Design review of the part built by this model. Coordinates are the model's own, in mm. A direction names the side the tool comes from. Coordinates: 2 decimals unless noted, no trailing zeros. One line per question, with ' | ' between items.
from build123d import *

# Parameters (mm, degrees)
SHELL1_T                                = -2.54
CUT_EXTRUDE2_DEPTH                      = 38.003022678
CIRPATTERN1_COUNT                       = 2
CIRPATTERN1_ANGLE                       = 90
BOSS_EXTRUDE3_DEPTH                     = 6.985
BOSS_EXTRUDE3_DEPTH_BACK                = 2.54
SKETCH13_R                              = 8.663884536
CBORE_FOR_M5_HEX_HEAD_BOLT2_D           = 4.5
CBORE_FOR_M5_HEX_HEAD_BOLT2_CBORE_D     = 7.5
CBORE_FOR_M5_HEX_HEAD_BOLT2_CBORE_DEPTH = 4


with BuildPart() as part:
    # Sketch1 → Revolve1 (revolve)
    with BuildSketch(Plane.XY, mode=Mode.PRIVATE) as revolve1_sk:
        with BuildLine():
            Line((0, 23.722851324), (5.5245, 23.722851324))
            ThreePointArc((5.5245, 23.722851324), (9.236535333, 23.238492745), (12.7, 21.817851324))
            Line((12.7, 21.817851324), (12.7, 20.547851324))
            Line((12.7, 20.547851324), (8.89, 20.547851324))
            add(Edge.make_bspline(
                [(8.89, 20.547851324), (8.84961008, 12.497906194), (9.741228483, 4.469234919), (9.525, -3.582148676)],
                knots=[0, 0, 0, 0, 1, 1, 1, 1], degree=3))
            Line((9.525, -3.582148676), (0, -3.582148676))
            Line((0, -3.582148676), (0, 23.722851324))
        make_face()
    revolve(revolve1_sk.sketch.rotate(Axis((0, 23.722851324, 0), (0, -1, 0)), 180), axis=Axis((0, 23.722851324, 0), (0, -1, 0)))

    # Shell1
    shell1_openings = [part.faces().sort_by_distance(p)[0] for p in [
        (0, -3.582148676, 0),
    ]]
    offset(amount=SHELL1_T, openings=shell1_openings, kind=Kind.INTERSECTION)

    # Sketch4 → Cut-Extrude2 (cut, through all)
    with BuildSketch(Plane.XY.offset(12.7)):
        with BuildLine():
            Line((0.9525, 12.292851324), (-0.9525, 12.292851324))
            add(Edge.make_bspline(
                [(-0.9525, 12.292851324), (-1.266575854, 4.327293664), (-2.2225, -3.582148676)],
                knots=[0, 0, 0, 1, 1, 1], degree=2))
            Line((-2.2225, -3.582148676), (2.2225, -3.582148676))
            add(Edge.make_bspline(
                [(0.9525, 12.292851324), (1.266575854, 4.327293664), (2.2225, -3.582148676)],
                knots=[0, 0, 0, 1, 1, 1], degree=2))
        make_face()
    cut_extrude2 = extrude(amount=-CUT_EXTRUDE2_DEPTH, mode=Mode.SUBTRACT)

    # CirPattern1: Cut-Extrude2 ×2 about axis
    cirpattern1_axis = Axis((0, 0, 0), (0, -1, 0))
    for i in range(1, CIRPATTERN1_COUNT):
        add(cut_extrude2.rotate(cirpattern1_axis, i * CIRPATTERN1_ANGLE / (CIRPATTERN1_COUNT - 1)), mode=Mode.SUBTRACT)

    # Sketch13 → Boss-Extrude3 (add, two sides: drawn at the far end of the back side and taken through both)
    with BuildSketch(Plane.XZ.offset(-20.547851324).offset(-BOSS_EXTRUDE3_DEPTH_BACK)):
        Circle(SKETCH13_R)
    extrude(amount=BOSS_EXTRUDE3_DEPTH + BOSS_EXTRUDE3_DEPTH_BACK)

    # CBORE for M5 Hex Head Bolt2 (through all)
    with Locations(Plane(origin=(0, 23.722851324, 0), x_dir=(-1, 0, 0), z_dir=(0, 1, 0))):
        with Locations((0, 0)):
            CounterBoreHole(CBORE_FOR_M5_HEX_HEAD_BOLT2_D / 2, CBORE_FOR_M5_HEX_HEAD_BOLT2_CBORE_D / 2, CBORE_FOR_M5_HEX_HEAD_BOLT2_CBORE_DEPTH)


solid = part.part
1. To check wall thickness, follow line 1 along Z through (x, y) = (0, 21.7); line 2 along Y through (x, z) = (2.75, 2.25); line 3 along Z through (x, y) = (0, 16.25). State the ranges of each line that lie inside material, in increasing order. Write a range as [from, to].
Answer sheet:
line 1: [-12.7, -3.75], [3.75, 12.7] | line 2: [13.56, 19.72] | line 3: [-8.95, -2.25], [2.25, 8.95]
2. Tool access review of faces 1 (the face through (9, 20.548, 3)), 2 (the face through (3.746, 21.751, 0.165)), 3 (the face through (0, 12.293, -8)), 4 (the face through (6, -3.582, 6)), 5 (the face through (8, 12.293, 0)): name each direction out of +Z, -Z, +X, -X, +Y, -Y from which nothing blocks a thin tool from reaching the whole face with its end or side.
Answer sheet:
face 1: none | face 2: +Y | face 3: +Z, -Z, -Y | face 4: +Z, -Z, +X, -X, -Y | face 5: +X, -X, -Y
3. Draft analysis for pull direction Z (two halves, no side actions). For faces 6 (the face through (0, 13.563, -3)), 7 (the face through (6, -3.582, -6)), 8 (the face through (-5.86, 21.174, 11.267)), state which applies: pulls with the +Z half, pulls with the -Z half, needs draft (parallel to the pull), parting line crosses it, or undercut.
Answer sheet:
face 6: undercut | face 7: needs draft | face 8: parting line crosses it
4. Take a section at A-A (y = 9). Count the separate pieces of the cut face and the enclosed holes in it, then the cut area to 3 significant figures.
Answer sheet:
separate pieces: 4 | enclosed holes: 0 | area: 105 mm^2
5. Insertion check: pin 1 Ø4 at (x, y) = (2.5, -0.5) entering from -Z; pin 2 Ø1 at (x, z) = (-7, 0) entering from -Y; pin 3 Ø4 at (x, y) = (9, 11.5) entering from -Z. Each pin has a flat end and moves straight along its axis. Give the tip position at first contact, or say it passes through.
Answer sheet:
pin 1: z = -9.39 | pin 2: y = 12.29 | pin 3: z = -5.87
